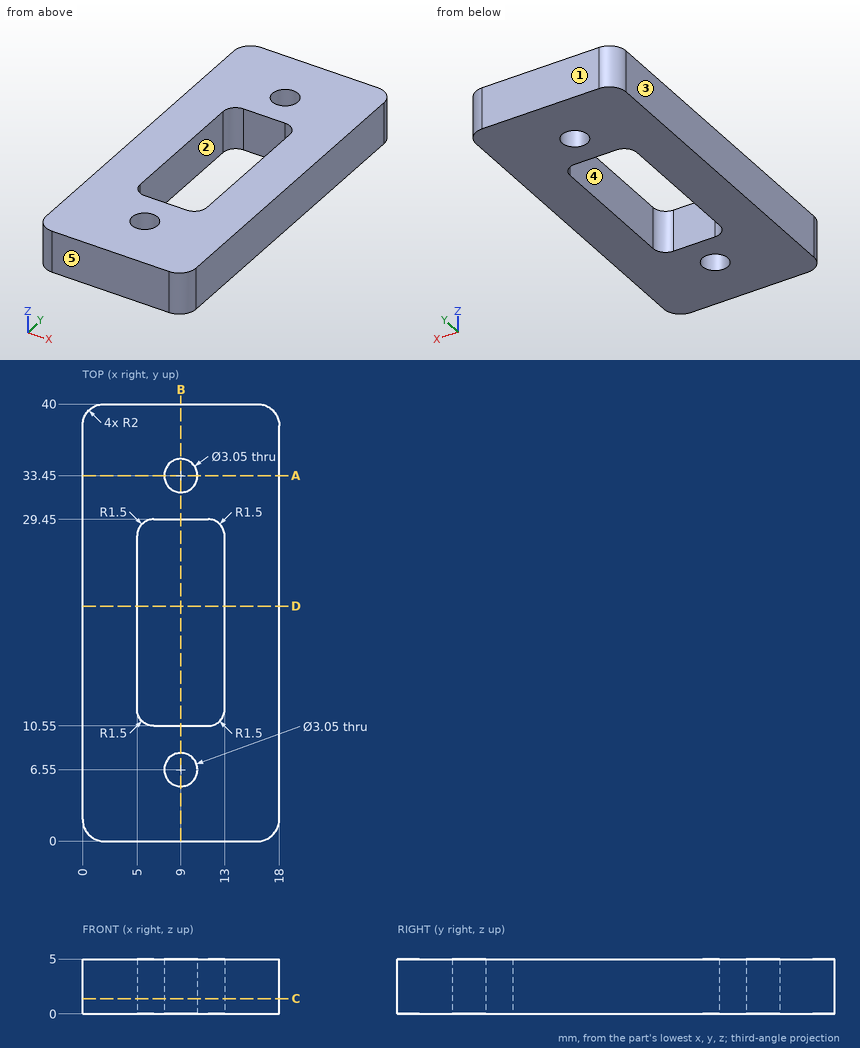
Study the drawing (mm; zero at the part's minimum x, y, z) and answer. A direction names the side the tool comes from. Round coordinates to 2 decimals unless told otherwise and drop trailing zeros. Write each loop counter-clockwise with the first axis right and the second up, starting at its lowest first coordinate (ties: lowest second). Pieces come first, ordered by that corner, then holes. Notation, with made-up numbers: (51, 17) - (83, 17) arc R26 ccw to (83, 44) - close; hole circle Ø10 at (68.25, 45.5). An arc over 180 degrees is marked (long way). Return JSON: item names as keys, results as strings. Group by question number.
Q1. The part is cut by section B-B on x = 9. Write down the section's boundary in (y, z) (3 decimals).
Q2. The part is cut by section D-D on y = 21.5. Write down the section's boundary in (x, z).
Q3. This flat-tipped pin is pushed along its axis until it touches: pin 1 Ø2 at (x, y) = (15.5, 34.5) entering from -Z. Where does it stop, or does it pass through?
Q4. The part is cut by section C-C on z = 1.4. Write down the section's boundary in (x, y) (3 decimals).
Q5. The mould has two halves that part along Y. Classify the marked faces 1, 2 and 3: released by +Y, released by -Y, zero draft, split by the parting line, or undercut.
Q6. For the marked faces 4 and 5, determine the directions among +Z, -Z, +X, -X, +Y, -Y from which every point of the face is accessible in a straight line to the end or side of a thin tool.
Q7. The part is cut by section A-A on y = 33.45. Write down the section's boundary in (x, z) (3 decimals), then the cut area to 4 significant figures.
Q8. Find the intervals of material crossed by L1, parallel to Y at x = 9, z = 2.95 (3 decimals); L2, parallel to Y at x = 11, z = 1.4; L3, parallel to X at y = 19, z = 4.4, in increasing order.
Solved:
{
 "1": {"outline": "(0, 0) - (5.025, 0) - (5.025, 5) - (0, 5) - close; (8.075, 0) - (10.55, 0) - (10.55, 5) - (8.075, 5) - close; (29.45, 0) - (31.925, 0) - (31.925, 5) - (29.45, 5) - close; (34.975, 0) - (40, 0) - (40, 5) - (34.975, 5) - close"},
 "2": {"outline": "(0, 0) - (5, 0) - (5, 5) - (0, 5) - close; (13, 0) - (18, 0) - (18, 5) - (13, 5) - close"},
 "3": {"pin 1": "z = 0"},
 "4": {"outline": "(0, 2) arc R2 ccw to (2, 0) - (16, 0) arc R2 ccw to (18, 2) - (18, 38) arc R2 ccw to (16, 40) - (2, 40) arc R2 ccw to (0, 38) - close; hole (5, 12.05) arc R1.5 ccw to (6.5, 10.55) - (11.5, 10.55) arc R1.5 ccw to (13, 12.05) - (13, 27.95) arc R1.5 ccw to (11.5, 29.45) - (6.5, 29.45) arc R1.5 ccw to (5, 27.95) - close; hole circle Ø3.05 at (9, 6.55); hole circle Ø3.05 at (9, 33.45)"},
 "5": {"face 1": "released by +Y", "face 2": "undercut", "face 3": "zero draft"},
 "6": {"face 4": "+Z, -Z", "face 5": "+Z, -Z, +X, -X, -Y"},
 "7": {"outline": "(0, 0) - (7.475, 0) - (7.475, 5) - (0, 5) - close; (10.525, 0) - (18, 0) - (18, 5) - (10.525, 5) - close", "area": "74.75 mm²"},
 "8": {"L1": "0 to 5.025, 8.075 to 10.55, 29.45 to 31.925, 34.975 to 40", "L2": "0 to 10.55, 29.45 to 40", "L3": "0 to 5, 13 to 18"}
}
